from build123d import *

# Parameters (mm, degrees)
SKETCH1_W           = 84.8
SKETCH1_H           = 165
SKETCH1_R           = 13.4
SKETCH1_R_2         = 4.925
BOSS_EXTRUDE1_DEPTH = 1.75
SKETCH1_3_W         = 84.8
SKETCH1_3_H         = 165
SKETCH1_3_R         = 13.4
BOSS_EXTRUDE2_DEPTH = 10
BOSS_EXTRUDE3_START = -24
SKETCH1_4_W         = 84.8
SKETCH1_4_H         = 165
SKETCH1_4_R         = 13.4
BOSS_EXTRUDE3_DEPTH = 24
DRAFT1_ANGLE        = 15


with BuildPart() as part:
    # Sketch1 → Boss-Extrude1 (new, symmetric)
    # profile 1 of 3: a face of its own
    with BuildSketch(Plane(origin=(0, 0, 0), x_dir=(1, 0, 0), z_dir=(0, 1, 0))):
        Rectangle(SKETCH1_W, SKETCH1_H)
        with Locations((-20, 0)):
            Circle(SKETCH1_R, mode=Mode.SUBTRACT)
        with Locations((20, 0)):
            Circle(SKETCH1_R, mode=Mode.SUBTRACT)
    # profile 2 of 3: a face of its own
    with BuildSketch(Plane(origin=(0, 0, 0), x_dir=(1, 0, 0), z_dir=(0, 1, 0))):
        with Locations((-20, 0)):
            Circle(SKETCH1_R)
        with Locations(Location((-20, 0, 0), (0, 0, 270))):
            Circle(SKETCH1_R_2, mode=Mode.SUBTRACT)
    # profile 3 of 3: a face of its own
    with BuildSketch(Plane(origin=(0, 0, 0), x_dir=(1, 0, 0), z_dir=(0, 1, 0))):
        with Locations((20, 0)):
            Circle(SKETCH1_R)
        with Locations(Location((20, 0, 0), (0, 0, 270))):
            Circle(SKETCH1_R_2, mode=Mode.SUBTRACT)
    extrude(amount=BOSS_EXTRUDE1_DEPTH, both=True)

    # Sketch1_3 → Boss-Extrude2 (add)
    with BuildSketch(Plane(origin=(0, 0, 0), x_dir=(1, 0, 0), z_dir=(0, 1, 0))):
        Rectangle(SKETCH1_3_W, SKETCH1_3_H)
        with Locations(Location((-20, 0, 0), (0, 0, 270))):
            Circle(SKETCH1_3_R, mode=Mode.SUBTRACT)
        with Locations(Location((20, 0, 0), (0, 0, 270))):
            Circle(SKETCH1_3_R, mode=Mode.SUBTRACT)
    extrude(amount=BOSS_EXTRUDE2_DEPTH)

    # Sketch1_4 → Boss-Extrude3 (add)
    with BuildSketch(Plane(origin=(0, 0, 0), x_dir=(1, 0, 0), z_dir=(0, 1, 0)).offset(BOSS_EXTRUDE3_START)):
        Rectangle(SKETCH1_4_W, SKETCH1_4_H)
        with Locations(Location((-20, 0, 0), (0, 0, 270))):
            Circle(SKETCH1_4_R, mode=Mode.SUBTRACT)
        with Locations(Location((20, 0, 0), (0, 0, 270))):
            Circle(SKETCH1_4_R, mode=Mode.SUBTRACT)
    extrude(amount=BOSS_EXTRUDE3_DEPTH)

    # Sketch3 → Cut-Revolve1 (revolve, cut)
    with BuildSketch(Plane(origin=(0, -12, 0), x_dir=(1, 0, 0), z_dir=(0, 1, 0)), mode=Mode.PRIVATE) as cut_revolve1_sk:
        Polygon((-6.25, -82.5), (-6.25, -76.5), (-5.25, -76.5), (-5.25, -61.5), (-4.05, -61.5), (-4.05, -47.5), (0, -47.5), (0, -82.5), align=None)
    cut_revolve1 = revolve(cut_revolve1_sk.sketch.rotate(Axis((0, -12, 82.5), (0, 0, -1)), 180), axis=Axis((0, -12, 82.5), (0, 0, -1)), mode=Mode.SUBTRACT)

    # Mirror1: Cut-Revolve1 across plane
    add(cut_revolve1.mirror(Plane.XY), mode=Mode.SUBTRACT)

    # Draft1
    draft1_faces = [part.faces().sort_by_distance(p)[0] for p in [
        (-20, 5.875, -13.4),
        (20, 5.875, -13.4),
    ]]
    draft(draft1_faces, Plane.ZX.offset(1.75), DRAFT1_ANGLE)


solid = part.part
Build history of the part. All positions in model axes, mm. A direction names the side the tool comes from. Round coordinates to 2 decimals unless told otherwise and drop trailing zeros. Write each loop counter-clockwise with the first axis right and the second up, starting at its lowest first coordinate (ties: lowest second). Pieces come first, ordered by that corner, then holes. Notation, with made-up numbers: M 43.5,37.5 L 80.5,37.5 A18 cw 80.5,41.5 Z; hole C 25.5,14 d7. An arc over 180 degrees is marked long. Answer as a JSON object with one key per item and string values. Group by question number.
(1) Mould opens along X. For faces 5 (the cylindrical face through (2.82, -16.43, -68.9)), 6 (the flat face through (-1, -3, -82.5)), 7 (the flat face through (-42.4, -7, 1)) say: pulls with the +X half, pulls with the -X half, needs draft (parallel to the pull), parting line crosses it, or undercut.
(2) Which spindle directions (+Z, -Z, +X, -X, +Y, -Y) get a long thin tool onto all of the face, cutting with end or side? Do faces 1 (the flat face through (20, 1.75, 6)), 2 (the cylindrical face through (-1.355, -5.899, -79.458)), 3 (the cylindrical face through (-0.878, -8.046, 54.402)), 4 (the cylindrical face through (-33.081, -13.031, -2.905)). Say none if no direction does.
(3) Cut at C-C (y = -22). Give the cut face in (x, z).
(4) Cut at A-A (x = 20). Give the cut face in (y, z) (3 decimals), and give its area (3 significant figures).
(5) Cut at D-D (x = 0). Give the cut face in (y, z), and give its area (3 significant figures).
(6) Cut at B-B (z = 0). Give the cut face in (x, y) (3 decimals).
(7) Drill centre lines: L1, parallel to X at y = -15.75, z = 0; L2, parallel to X at y = 0, z = 0 (3 decimals); L3, parallel to Z at x = 20, y = -11. Where is each one in solid material? Low to high.
(8) Flat gauge pins, fed straight in: pin 1 (9 mm diameter, centred on x = -1, y = -12.5, fed in from +Z); pin 2 (8 mm diameter, centred on x = 20, z = 0, fed in from -Y); pin 3 (6 mm diameter, centred on x = 0.5, y = -13, fed in from +Z); pin 4 (24 mm diameter, centred on x = -20, z = 0, fed in from -Y). Where does each tip first touch, or does it go through?
Responses:
{
 "1": {"face 5": "undercut", "face 6": "needs draft", "face 7": "pulls with the -X half"},
 "2": {"face 1": "+Y", "face 2": "-Z", "face 3": "+Z", "face 4": "-Y"},
 "3": {"outline": "M -42.4,-82.5 L 42.4,-82.5 L 42.4,82.5 L -42.4,82.5 Z; hole C -20,0 d26.8; hole C 20,0 d26.8"},
 "4": {"outline": "M -24,-82.5 L 10,-82.5 L 10,-15.611 L 1.75,-13.4 L 1.75,-4.925 L -1.75,-4.925 L -1.75,-13.4 L -24,-13.4 Z; M -24,13.4 L -1.75,13.4 L -1.75,4.925 L 1.75,4.925 L 1.75,13.4 L 10,15.611 L 10,82.5 L -24,82.5 Z", "area": "4,740 mm2"},
 "5": {"outline": "M -24,-82.5 L -18.25,-82.5 L -18.25,-76.5 L -17.25,-76.5 L -17.25,-61.5 L -16.05,-61.5 L -16.05,-47.5 L -7.95,-47.5 L -7.95,-61.5 L -6.75,-61.5 L -6.75,-76.5 L -5.75,-76.5 L -5.75,-82.5 L 10,-82.5 L 10,82.5 L -5.75,82.5 L -5.75,76.5 L -6.75,76.5 L -6.75,61.5 L -7.95,61.5 L -7.95,47.5 L -16.05,47.5 L -16.05,61.5 L -17.25,61.5 L -17.25,76.5 L -18.25,76.5 L -18.25,82.5 L -24,82.5 Z", "area": "4,920 mm2"},
 "6": {"outline": "M -42.4,-24 L -33.4,-24 L -33.4,-1.75 L -24.925,-1.75 L -24.925,1.75 L -33.4,1.75 L -35.611,10 L -42.4,10 Z; M -15.075,-1.75 L -6.6,-1.75 L -6.6,-24 L 6.6,-24 L 6.6,-1.75 L 15.075,-1.75 L 15.075,1.75 L 6.6,1.75 L 4.389,10 L -4.389,10 L -6.6,1.75 L -15.075,1.75 Z; M 24.925,-1.75 L 33.4,-1.75 L 33.4,-24 L 42.4,-24 L 42.4,10 L 35.611,10 L 33.4,1.75 L 24.925,1.75 Z"},
 "7": {"L1": "x = -42.4 to -33.4, -6.6 to 6.6, 33.4 to 42.4", "L2": "x = -42.4 to -24.925, -15.075 to 15.075, 24.925 to 42.4", "L3": "z = -82.5 to -13.4, 13.4 to 82.5"},
 "8": {"pin 1": "stops at z = 76.5", "pin 2": "passes through", "pin 3": "stops at z = 61.5", "pin 4": "stops at y = -1.75"}
}
